Check sheet for the modelled part. Datum: model origin and axes. Units: mm. A direction names the side the tool comes from. Coordinates: 2 decimals unless noted, no trailing zeros. Write each loop counter-clockwise with the first axis right and the second up, starting at its lowest first coordinate (ties: lowest second). Pieces come first, ordered by that corner, then holes. Notation, with made-up numbers: M 20.25,-37 L 50.25,-37 A13 ccw 50.25,-21 Z; hole C 13,80 d2. An arc over 180 degrees is marked long. Answer as CSV lines item,"result".
Autodesk Inventor part; units mm, degrees
ref_plane "YZ Plane" through (0, 0, 0) normal (1, 0, 0) x (0, 1, 0)
ref_plane "XZ Plane" through (0, 0, 0) normal (0, 1, 0) x (-1, 0, 0)
ref_plane "XY Plane" through (0, 0, 0) normal (0, 0, 1) x (1, 0, 0)
sketch "Esboço1" plane through (0, 0, 0) normal (0, 0, 1) x (1, 0, 0)
  line L0 (0, 0) -> (0, 11)
  line L1 (0, 5) -> (-10.2862, 5) construction
  line L2 (0, 9.05) -> (6.4587, 9.05) construction
  line L3 (3.2294, 11) -> (3.2294, 8.5) construction
  line L4 (1.95, 8.4353) -> (1, 9.1471)
  line L5 (1.95, 6.85) -> (1.95, 8.4353)
  line L6 (1.45, 6.85) -> (1.95, 6.85)
  line L7 (1.45, 6.85) -> (1.45, 4.75)
  line L8 (0, 4.75) -> (6.1218, 4.75) construction
  line L9 (1.75, 4.75) -> (1.75, 0)
  line L10 (1.75, 4.75) -> (1.45, 4.75)
  line L11 (0, 11) -> (1, 11)
  line L12 (1, 11) -> (1, 9.1471)
  line L13 (0, 0) -> (1.75, 0)
  point P0 (0, 0)
  dimension "d17" = 1
  dimension "d24" = 1.95
  dimension "d25" = 1.75
  dimension "d26" = 2.1
  dimension "d27" = 1.45
revolve "Revolução1" add sketch "Esboço1" angle 360 about axis through (0, 0, 0) along (0, 1, 0)
properties part number "travaInternaRoda"
1) Section check B-B, the plane z = 0. Record the boundary of the cut face in (x, y), plus the area to 3 significant figures.
Answer key:
outline,"M -1.95,6.85 L -1.45,6.85 L -1.45,4.75 L -1.75,4.75 L -1.75,0 L 1.75,0 L 1.75,4.75 L 1.45,4.75 L 1.45,6.85 L 1.95,6.85 L 1.95,8.44 L 1,9.15 L 1,11 L -1,11 L -1,9.15 L -1.95,8.44 Z"
area,"34.7 mm2"
2) Section check D-D, the plane y = 7. Record the boundary of the cut face in (x, z), plus the area to 3 significant figures.
Answer key:
outline,"C 0,0 d3.9"
area,"11.9 mm2"
3) Section check C-C, the plane y = 1. Record the boundary of the cut face in (x, z), plus the area to 3 significant figures.
Answer key:
outline,"C 0,0 d3.5"
area,"9.62 mm2"
4) Thickness scan on line 1 along X through (y, z) = (7.5, -0.1); line 2 along Y through (x, z) = (1.7, 0.55); line 3 along Y through (x, z) = (-1.55, 0) (3 decimals). Record the ranges inside material, lowest first.
Answer key:
line 1,"x = -1.95 to 1.95"
line 2,"y = 6.85 to 8.56"
line 3,"y = 0 to 4.75, 6.85 to 8.735"
5) Tool access check on faces 4 (the face through (-1.437, 7.654, -1.318)), 5 (the face through (0, 10, -1)). Record the directions out of +Z, -Z, +X, -X, +Y, -Y that give a thin tool (end or side, any length) a straight path to the whole face; none if there is none.
Answer key:
face 4,"+Y, -Y"
face 5,"+Y"
6) Section check A-A, the plane x = 0. Record the boundary of the cut face in (y, z), plus the area to 3 significant figures.
Answer key:
outline,"M 0,-1.75 L 4.75,-1.75 L 4.75,-1.45 L 6.85,-1.45 L 6.85,-1.95 L 8.44,-1.95 L 9.15,-1 L 11,-1 L 11,1 L 9.15,1 L 8.44,1.95 L 6.85,1.95 L 6.85,1.45 L 4.75,1.45 L 4.75,1.75 L 0,1.75 Z"
area,"34.7 mm2"
7) Mould release check, pull along Y, two halves, no side actions. Record for faces 1 (the face through (0, 11, 0)), 2 (the face through (-1.45, 5.79, 0.06)), 3 (the face through (1.617, 2.342, -0.67)): pulls with the +Y half, pulls with the -Y half, needs draft (parallel to the pull), parting line crosses it, or undercut.
Answer key:
face 1,"pulls with the +Y half"
face 2,"undercut"
face 3,"needs draft"
